from build123d import *

# Parameters (mm, degrees)
PAD_DEPTH          = 10
SKETCH001_R        = 2.5
POCKET_DEPTH       = 5
POLARPATTERN_COUNT = 9


with BuildPart() as part:
    # Sketch → Pad (new body)
    with BuildSketch(Plane.XZ):
        with BuildLine():
            ThreePointArc((-94.682835, 147.173913), (0, -175), (94.682835, 147.173913))
            ThreePointArc((52.148431, 29.673913), (94.028813, 80.962046), (94.682835, 147.173913))
            ThreePointArc((37.712362, -46.666667), (58.955166, -11.148473), (52.148431, 29.673913))
            ThreePointArc((-37.712362, -46.666667), (0, -100), (37.712362, -46.666667))
            ThreePointArc((-52.148431, 29.673913), (-58.955166, -11.148473), (-37.712362, -46.666667))
            ThreePointArc((-94.682835, 147.173913), (-94.028813, 80.962046), (-52.148431, 29.673913))
        make_face()
    extrude(amount=PAD_DEPTH)

    # Sketch001 (on Face8 of Pad) → Pocket (cut)
    with BuildSketch(Plane.XZ.offset(10)):
        with Locations((0, 147.864497)):
            Circle(SKETCH001_R)
    pocket = extrude(amount=-POCKET_DEPTH, mode=Mode.SUBTRACT)

    # PolarPattern: Pocket ×9 about axis
    polarpattern_axis = Axis((0, -10, 0), (0, -1, 0))
    for i in range(1, POLARPATTERN_COUNT):
        add(pocket.rotate(polarpattern_axis, i * 360 / POLARPATTERN_COUNT), mode=Mode.SUBTRACT)


solid = part.part
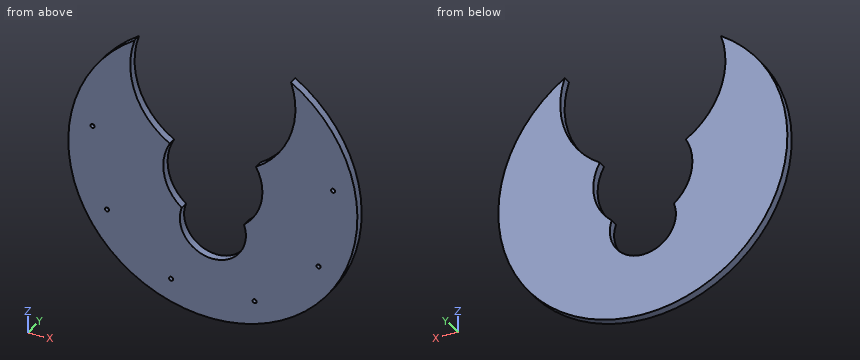
The listing builds one solid part. Answer for the finished solid, in the listing's coordinates (mm). Round coordinates to 2 decimals unless told otherwise and drop trailing zeros. Write each loop counter-clockwise with the first axis right and the second up, starting at its lowest first coordinate (ties: lowest second). Pieces come first, ordered by that corner, then holes. Notation, with made-up numbers: M 4.25,-4.5 L 56.25,-4.5 A29 ccw 56.25,34.5 Z; hole C -37.75,-4.5 d3. An arc over 180 degrees is marked long. Write each question's results on one line, items separated by ' | '. Start each with the question number.
Item 1: Find section B-B on y = -7.5. Write down the section's boundary in (x, z), and give its area (3 significant figures).
Item 2: Find section A-A on z = 0. Write down the section's boundary in (x, y).
Item 3: Straight lines are drawn through the part: probe 1 along X at (y, z) = (-8.5, -83.5); probe 2 along X at (y, z) = (-6, 117.5); probe 3 along Z at (x, y) = (-115, -1.5). For each, find the intervals that lie inside material, in ascending order.
Item 4: Find section C-C on x = 0. Write down the section's boundary in (y, z), and give its area (3 significant figures).
Item 5: Find section D-D on z = 48.5. Write down the section's boundary in (x, y), and give its area (3 significant figures).
Item 6: Given pin 1 Ø1.5 at (x, z) = (51.5, -138.5) entering from -Y; pin 2 Ø1 at (x, y) = (45.5, -1.5) entering from +Z; pin 3 Ø1 at (y, z) = (-5, -20.5) entering from -X, each flat-ended and moving along its own axis, determine where each tip first touches the part or whether it passes through.
Answer block:
1) outline: M -94.68,147.17 A175 ccw long 94.68,147.17 A100 cw 52.15,29.67 A60 cw 37.71,-46.67 A40 cw long -37.71,-46.67 A60 cw -52.15,29.67 A100 cw Z; hole C -145.62,25.68 d5; hole C -128.05,-73.93 d5; hole C -50.57,-138.95 d5; hole C 50.57,-138.95 d5; hole C 128.05,-73.93 d5; hole C 145.62,25.68 d5 | area: 59,600 mm²
2) outline: M -175,-10 L -60,-10 L -60,0 L -175,0 Z; M 60,-10 L 175,-10 L 175,0 L 60,0 Z
3) probe 1: x = -153.79 to -32.37, 32.37 to 153.79 | probe 2: x = -129.69 to -99.97, 99.97 to 129.69 | probe 3: z = -131.91 to 131.91
4) outline: M -10,-175 L 0,-175 L 0,-100 L -10,-100 Z | area: 750 mm²
5) outline: M -168.15,-10 L -74.68,-10 L -74.68,0 L -168.15,0 Z; M 74.68,-10 L 168.15,-10 L 168.15,0 L 74.68,0 Z | area: 1,870 mm²
6) pin 1: stops at y = -5 | pin 2: stops at z = -38.52 | pin 3: stops at x = -173.85
